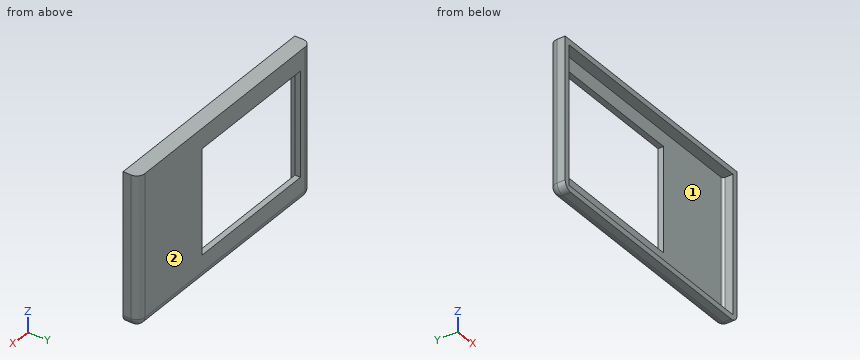
```python
from build123d import *

# Parameters (mm, degrees)
SKETCH1_W           = 300
SKETCH1_H           = 187
BOSS_EXTRUDE1_DEPTH = 20
FILLET1_R           = 10
FILLET2_R           = 10
SHELL2_T            = -7
SKETCH2_W           = 172
SKETCH2_H           = 131
CUT_EXTRUDE2_DEPTH  = 7
FILLET3_R           = 10


with BuildPart() as part:
    # Sketch1 → Boss-Extrude1 (new body)
    with BuildSketch(Plane(origin=(0, 0, 0), x_dir=(1, 0, 0), z_dir=(0, 1, 0))):
        with Locations((71.737321437, -61.518699121)):
            Rectangle(SKETCH1_W, SKETCH1_H)
    extrude(amount=BOSS_EXTRUDE1_DEPTH)

    # Fillet1
    fillet1_edges = [part.edges().sort_by_distance(p)[0] for p in [
        (-78.262678563, 20, 61.518699121),
    ]]
    fillet(fillet1_edges, radius=FILLET1_R)

    # Fillet2
    fillet2_edges = [part.edges().sort_by_distance(p)[0] for p in [
        (221.737321437, 20, 61.518699121),
    ]]
    fillet(fillet2_edges, radius=FILLET2_R)

    # Shell2
    shell2_openings = [part.faces().sort_by_distance(p)[0] for p in [
        (71.737321437, 0, 61.518699121),
    ]]
    offset(amount=SHELL2_T, openings=shell2_openings, kind=Kind.INTERSECTION)

    # Sketch2 → Cut-Extrude2 (cut)
    with BuildSketch(Plane(origin=(0, 20, 0), x_dir=(1, 0, 0), z_dir=(0, 1, 0))):
        with Locations((25.737321437, -64.518699121)):
            Rectangle(SKETCH2_W, SKETCH2_H)
    extrude(amount=-CUT_EXTRUDE2_DEPTH, mode=Mode.SUBTRACT)

    # Fillet3
    fillet3_edges = [part.edges().sort_by_distance(p)[0] for p in [
        (71.737321437, 20, -31.981300879),
        (-78.262678563, 5, -31.981300879),
        (-75.333746375, 17.071067812, -31.981300879),
        (221.737321437, 5, -31.981300879),
        (218.808389249, 17.071067812, -31.981300879),
    ]]
    fillet(fillet3_edges, radius=FILLET3_R)


solid = part.part
```
Geometry: final body of the model. Coordinates: model frame, mm. Face numbers are marked on the shaded views. Give positions to 0.01 mm unless a question says otherwise; leave off trailing zeros. Write each loop counter-clockwise with the first axis right and the second up, starting at its lowest first coordinate (ties: lowest second). Pieces come first, ordered by that corner, then holes.
1. Line query: probe 1 along Z at (x, y) = (34, 3); probe 2 along X at (y, z) = (4.5, 140); probe 3 along Y at (x, z) = (134, 133). Output: solid intervals per line, ascending.
2. Section query B-B, the plane y = 6.25. Return loops of the section in (x, z), then the cut area to 3 significant figures.
3. Draft query along X for the marked faces 1 and 2. Return one class per face: released by +X, released by -X, zero draft, split by the parting line, or undercut.
4. Pin query (flat end, axial travel): P1, Ø3.5, axis at y = 16.5, z = 96, coming from the +X side; P2, Ø7.5, axis at x = 14, y = 18, coming from the -Z side; P3, Ø1, axis at x = 157, y = 14, coming from the -Z side. Return the tip coordinate at first contact, or that it passes through.
5. Section query D-D, the plane x = 161. Return loops of the section in (y, z), then the cut area to 3 significant figures.
6. Section query A-A, the plane x = -38.5. Return loops of the section in (y, z), then the cut area to 3 significant figures.
7. Section query C-C, the plane z = 41. Return loops of the section in (x, y), then the cut area to 3 significant figures.
Computed:
1. probe 1: z = -31.98 to -24.98, 148.02 to 155.02
1. probe 2: x = -78.26 to -71.26, 214.74 to 221.74
1. probe 3: y = 13 to 20
2. outline: (-78.26, -21.98) arc R10 ccw to (-68.26, -31.98) - (211.74, -31.98) arc R10 ccw to (221.74, -21.98) - (221.74, 155.02) - (-78.26, 155.02) - close; hole (-71.26, -24.98) - (214.74, -24.98) - (214.74, 148.02) - (-71.26, 148.02) - close
2. area: 6,580 mm2
3. face 1: undercut
3. face 2: zero draft
4. P1: stops at x = 220.54
4. P2: stops at z = -31.03
4. P3: stops at z = -31.35
5. outline: (0, -31.98) - (10, -31.98) arc R10 ccw to (20, -21.98) - (20, 155.02) - (0, 155.02) - (0, 148.02) - (13, 148.02) - (13, -24.98) - (0, -24.98) - close
5. area: 1,470 mm2
6. outline: (0, -31.98) - (10, -31.98) arc R10 ccw to (20, -21.98) - (20, -0.98) - (13, -0.98) - (13, -24.98) - (0, -24.98) - close; (0, 148.02) - (13, 148.02) - (13, 130.02) - (20, 130.02) - (20, 155.02) - (0, 155.02) - close
6. area: 553 mm2
7. outline: (-78.26, 0) - (-71.26, 0) - (-71.26, 10) arc R3 cw to (-68.26, 13) - (-60.26, 13) - (-60.26, 20) - (-68.26, 20) arc R10 ccw to (-78.26, 10) - close; (111.74, 13) - (211.74, 13) arc R3 cw to (214.74, 10) - (214.74, 0) - (221.74, 0) - (221.74, 10) arc R10 ccw to (211.74, 20) - (111.74, 20) - close
7. area: 1,040 mm2
